Source: CAD feature listing. Evaluate the final solid. Frame: model axes, mm. Coordinates: 2 decimals unless noted, no trailing zeros. Loops run counter-clockwise (first coordinate to the right, second up) from the corner with the lowest first, then second, coordinate; pieces in that order, holes last. Notation, with made-up numbers: (41.5, 86) - (57.5, 86) arc R16 ccw to (57.5, 111) - close; hole circle Ø2 at (42, 73.5). An arc over 180 degrees is marked (long way). Write item = value, one per line. Start each with the question number.
from build123d import *

# Parameters (mm, degrees)
BASPROSKE_W        = 10
BASPROSKE_H        = 6
TOOTHCUT_DEPTH     = 14.114877049
TEETHCUTS_COUNT    = 10
TEETHCUTS_ANGLE    = 324
BORSKE_R           = 0.4
BORE_DEPTH         = 50.0000508
SKETCH1_R          = 0.4
CUT_EXTRUDE1_DEPTH = 13.998849476


with BuildPart() as part:
    # BasProSke → Base-Revolve (revolve)
    with BuildSketch(Plane(origin=(0, 0, 0), x_dir=(1, 0, 0), z_dir=(0, 1, 0)), mode=Mode.PRIVATE) as base_revolve_sk:
        with Locations((5, 3)):
            Rectangle(BASPROSKE_W, BASPROSKE_H)
    revolve(base_revolve_sk.sketch.rotate(Axis((-10, 0, 0), (1, 0, 0)), 180), axis=Axis((-10, 0, 0), (1, 0, 0)))

    # TooCutSke → ToothCut (cut, through all)
    with BuildSketch(Plane(origin=(0, 0, 0), x_dir=(0, 0, -1), z_dir=(1, 0, 0))):
        with BuildLine():
            ThreePointArc((0.59278292, 3.701838653), (0, 3.749), (-0.59278292, 3.701838653))
            ThreePointArc((-0.59278292, 3.701838653), (-0.846593509, 4.924114224), (-1.775771316, 5.757784417))
            ThreePointArc((-1.775771316, 5.757784417), (0, 6.0254), (1.775771316, 5.757784417))
            ThreePointArc((1.775771316, 5.757784417), (0.846593509, 4.924114224), (0.59278292, 3.701838653))
        make_face()
    toothcut = extrude(amount=TOOTHCUT_DEPTH, mode=Mode.SUBTRACT)

    # TeethCuts: ToothCut ×10 about axis
    teethcuts_axis = Axis((-10, 0, 0), (1, 0, 0))
    for i in range(1, TEETHCUTS_COUNT):
        add(toothcut.rotate(teethcuts_axis, i * TEETHCUTS_ANGLE / (TEETHCUTS_COUNT - 1)), mode=Mode.SUBTRACT)

    # BorSke → Bore (cut, symmetric)
    with BuildSketch(Plane(origin=(0, 0, 0), x_dir=(0, 0, -1), z_dir=(1, 0, 0))):
        with Locations(Location((0, 0, 0), (0, 0, 180))):
            Circle(BORSKE_R)
    extrude(amount=BORE_DEPTH, both=True, mode=Mode.SUBTRACT)

    # Sketch1 → Cut-Extrude1 (cut, through all)
    with BuildSketch(Plane(origin=(10, 0, 0), x_dir=(0, 0, -1), z_dir=(1, 0, 0))):
        with BuildLine():
            ThreePointArc((-1.708617862, 1.825), (-2.5, 0), (-1.708617862, -1.825))
            Line((-1.708617862, -1.825), (1.708617862, -1.825))
            ThreePointArc((1.708617862, -1.825), (2.293637358, -0.994599252), (2.5, 0))
            ThreePointArc((2.5, 0), (2.293637358, 0.994599252), (1.708617862, 1.825))
            Line((1.708617862, 1.825), (-1.708617862, 1.825))
        make_face()
        Circle(SKETCH1_R, mode=Mode.SUBTRACT)
    extrude(amount=-CUT_EXTRUDE1_DEPTH, mode=Mode.SUBTRACT)


solid = part.part
Item 1: Cut plane B-B (y = 1). Return the cut outline in (x, z).
Item 2: First-contact query: pin 1 (5 mm diameter, centred on x = 3.5, y = 4, fed in from -Z); pin 2 (6 mm diameter, centred on y = 4, z = -3.5, fed in from -X); pin 3 (4 mm diameter, centred on x = 4, z = -0.5, fed in from -Y); pin 4 (2 mm diameter, centred on x = 8, y = 4, fed in from +Z). Flat tips, straight axial feed; report the tip coordinate or a pass-through.
Item 3: Cut plane A-A (y = -4.5). Return the cut outline in (x, z).
Item 4: Material intervals for L1, parallel to Z at x = 2, y = 0; L2, parallel to Z at x = 6.75, y = -2.75; L3, parallel to Z at x = 4.5, y = 3.5, sorted ascending. Write a range as [from, to].
Item 5: Cut plane C-C (y = -2). Return the cut outline in (x, z).
Responses:
q1.outline = (0, -3.61) - (10, -3.61) - (10, -2.29) - (0, -2.29) - close; (0, 2.29) - (10, 2.29) - (10, 3.61) - (0, 3.61) - close
q2.pin_1 = -4.92
q2.pin_2 = 0
q2.pin_3 = -5.74
q2.pin_4 = 4.92
q3.outline = (0, -2.21) - (10, -2.21) - (10, -0.66) - (0, -0.66) - close; (0, 0.66) - (10, 0.66) - (10, 2.21) - (0, 2.21) - close
q4.L1 = [-6, -2.5], [2.5, 6]
q4.L2 = [-4.71, -2.72], [-2.55, 2.55], [2.72, 4.71]
q4.L3 = [-4.87, -3.61], [-1.83, 1.83], [3.61, 4.87]
q5.outline = (0, -4.04) - (10, -4.04) - (10, 4.04) - (0, 4.04) - close
